Source: three-view drawing plus pictorial views. Frame: mm from the lowest corner of the part. Give positions to 0.01 mm unless a question says otherwise; leave off trailing zeros. Order: outer loops, then holes, each group sorted by start corner. A loop starts at its lowest first (then second) coordinate and runs counter-clockwise, first axis right, second up. Notation, with made-up numbers: (10, 63) -> (57, 63) arc R20 cw to (57, 102) -> close; hole circle Ø2 at (40.5, 16). An arc over 180 degrees is marked (long way). Write item = value, one per line.
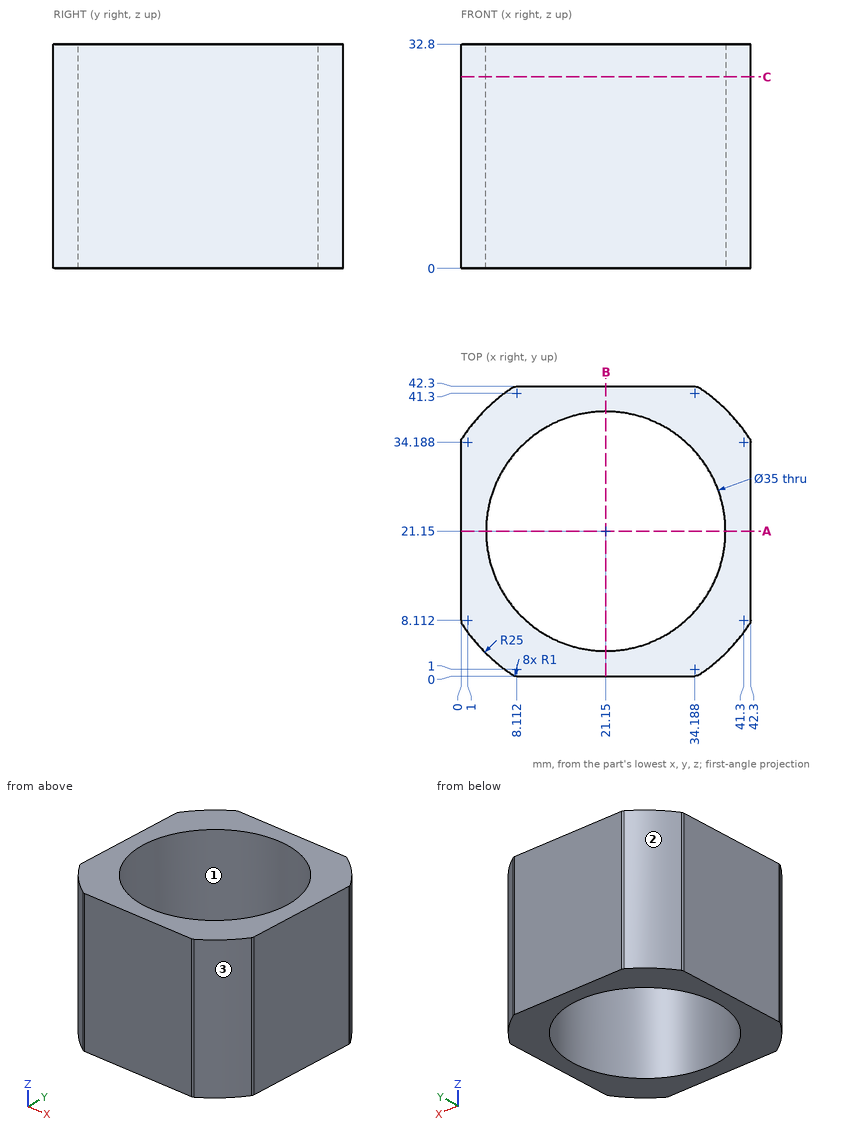
1) First-contact query: P1, Ø1, axis at y = 35.5, z = 21, coming from the +X side. Flat tip, straight axial feed; report the tip coordinate or a pass-through.
Check sheet entries:
P1 = 41.96
2) Mould query, pull axis X, two halves, no side actions, for the marked faces 1, 2 and 3. Classes: +X half, -X half, draft (parallel to the pull), parting line (faces both ways), or undercut.
Check sheet entries:
face_1 = undercut
face_2 = -X half
face_3 = +X half
3) Line query: line 1 (Y direction, x = 21.15, z = 20); line 2 (X direction, y = 27, z = 8). Output: solid intervals per line, ascending. Write a range as from..to.
Check sheet entries:
line_1 = 0..3.65, 38.65..42.3
line_2 = 0..4.66, 37.64..42.3
4) Section query C-C (z = 28). Output: boundary loops of the cut face in (x, y), plus the area to 3 significant figures.
Check sheet entries:
outline = (0, 8.11) arc R1 ccw to (0.16, 7.57) arc R25 ccw to (7.57, 0.16) arc R1 ccw to (8.11, 0) -> (34.19, 0) arc R1 ccw to (34.73, 0.16) arc R25 ccw to (42.14, 7.57) arc R1 ccw to (42.3, 8.11) -> (42.3, 34.19) arc R1 ccw to (42.14, 34.73) arc R25 ccw to (34.73, 42.14) arc R1 ccw to (34.19, 42.3) -> (8.11, 42.3) arc R1 ccw to (7.57, 42.14) arc R25 ccw to (0.16, 34.73) arc R1 ccw to (0, 34.19) -> close; hole circle Ø35 at (21.15, 21.15)
area = 723 mm²
5) Section query A-A (y = 21.15). Output: boundary loops of the cut face in (x, z).
Check sheet entries:
outline = (0, 0) -> (3.65, 0) -> (3.65, 32.8) -> (0, 32.8) -> close; (38.65, 0) -> (42.3, 0) -> (42.3, 32.8) -> (38.65, 32.8) -> close
